The listing builds one solid part. Answer for the finished solid, in the listing's coordinates (mm). A direction names the side the tool comes from. Coordinates: 2 decimals unless noted, no trailing zeros. Use one line per item in the form item = value. Start each with the question number.
Item 1: Consider line 1 along Y through (x, z) = (0, 11.9); line 2 along X through (y, z) = (0, 11.45). Determine where each line is inside the solid, lowest interval first. Write a range as [from, to].
Item 2: Each of these flat-tipped pins is pushed along its axis until it touches: pin 1 Ø4 at (x, z) = (30.5, 10.5) entering from +Y; pin 2 Ø1 at (x, z) = (33, 11.5) entering from -Y; pin 3 Ø2 at (y, z) = (13, 5) entering from -X. Where does it stop, or does it pass through?
Item 3: The mould has two halves that part along Z. Classify faces 4 (the cylindrical face through (56, -12, 12)), 5 (the conical face through (48.94, -10.868, 10.304)), 6 (the cylindrical face through (53.25, -11.82, 5.28)), 7 (the flat face through (-40, 35, 0)): released by +Z, released by -Z, zero draft, split by the parting line, or undercut.
Item 4: A tool of negligible diameter and unlimited length cuts with its end or side. For faces 1 (the flat face through (-46.2, -29.5, 2.786)), 2 (the flat face through (-45, -29, 12.071)), 3 (the flat face through (-48.4, -30.9, 13)), from which of +Z, -Z, +X, -X, +Y, -Y can it reach the whole face along a straight path? Write none if from no direction.
from build123d import *


with BuildPart() as part:
    # 스케치1 → 회전1 (revolve)
    with BuildSketch(Plane(origin=(0, 0, 0), x_dir=(0, 0, -1), z_dir=(1, 0, 0))):
        with BuildLine():
            Line((-10.214285714, 57.272727273), (-2.785714286, 56.363636364))
            Line((-2.785714286, 56.363636364), (-2.785714286, 54.545454545))
            Line((-2.785714286, 54.545454545), (-7.711122642, 54.545454545))
            ThreePointArc((-7.711122642, 54.545454545), (-9.285714286, 55.454545455), (-10.860305929, 54.545454545))
            Line((-10.860305929, 54.545454545), (-12.071428571, 54.545454545))
            Line((-12.071428571, 54.545454545), (-12.071428571, 52.727272727))
            Line((-12.071428571, 52.727272727), (-10.214285714, 50))
            Line((-10.214285714, 50), (-6.5, 51.818181818))
            Line((-6.5, 51.818181818), (-3.796015479, 52.196361472))
            Line((-3.796015479, 52.196361472), (-1.599654007, 50))
            Line((-1.599654007, 50), (-1.181818182, 50.417835825))
            Line((-1.181818182, 50.417835825), (-1.924421913, 52.458122809))
            Line((-1.924421913, 52.458122809), (0, 52.727272727))
            Line((0, 52.727272727), (0, 59.071428571))
            Line((0, 59.071428571), (-0.928571429, 60))
            Line((-0.928571429, 60), (-12.071428571, 60))
            Line((-12.071428571, 60), (-13, 59.071428571))
            Line((-13, 59.071428571), (-13, 57.272727273))
            Line((-13, 57.272727273), (-10.214285714, 57.272727273))
        make_face()
    revolve(axis=Axis((0, 0, 0), (0, 0, 1)))


solid = part.part
Response:
q1.line_1 = [-60, -57.27], [-54.55, -52.48], [52.48, 54.55], [57.27, 60]
q1.line_2 = [-60, -57.27], [-54.55, -51.81], [51.81, 54.55], [57.27, 60]
q2.pin_1 = 52.8
q2.pin_2 = -50.44
q2.pin_3 = -58.79
q3.face_4 = zero draft
q3.face_5 = released by +Z
q3.face_6 = undercut
q3.face_7 = released by -Z
q4.face_1 = none
q4.face_2 = +Z
q4.face_3 = +Z, +X, -X, +Y, -Y
